Print and shaded views of the part. All mm, measured from the part's lowest x, y and z. Give positions to 0.01 mm unless a question says otherwise; leave off trailing zeros. Loops run counter-clockwise (first coordinate to the right, second up) from the corner with the lowest first, then second, coordinate; pieces in that order, holes last. Notation, with made-up numbers: (78, 34) - (116, 34) arc R19 ccw to (116, 50) - close; hole circle Ø2 at (34, 61). An arc over 180 degrees is marked (long way). Return JSON: item names as keys, results as strings.
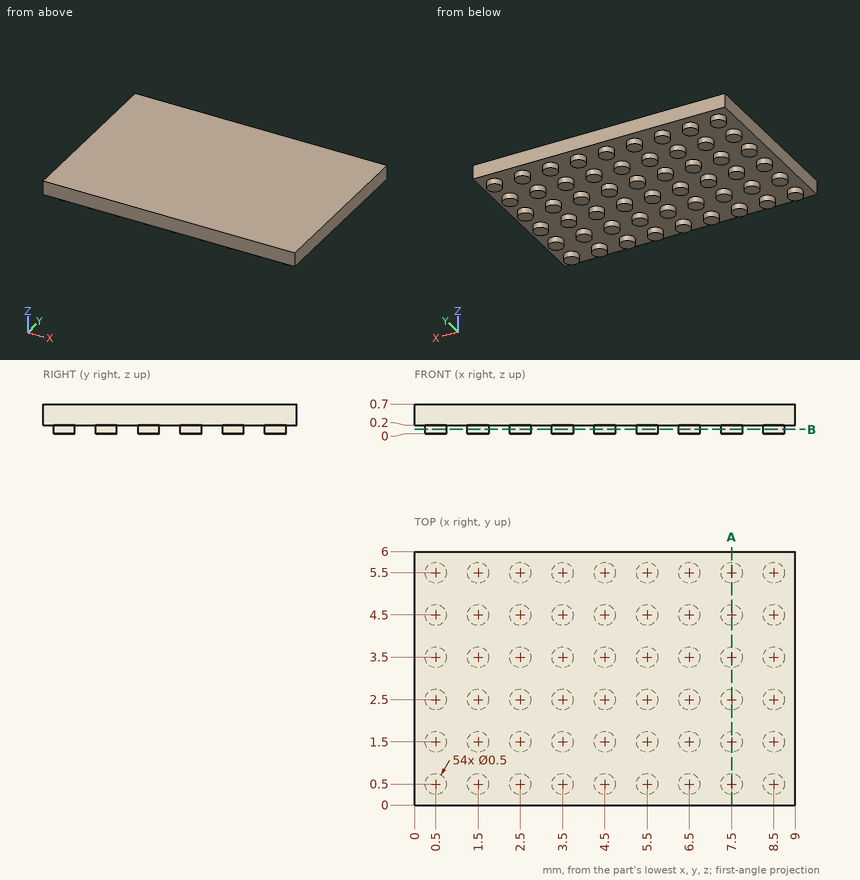
1. Cut at B-B, the plane z = 0.1. Give the number of separate pieces and of enclosed holes in the cut face, plus the area to 3 significant figures.
Values follow:
{"separate pieces": "54", "enclosed holes": "0", "area": "10.6 mm²"}
2. Drill centre lines: probe 1 along Y at (x, z) = (0.5, 0.1); probe 2 along Z at (x, y) = (5, 5.5). Where is each one in solid material? Low to high.
Values follow:
{"probe 1": "y = 0.25 to 0.75, 1.25 to 1.75, 2.25 to 2.75, 3.25 to 3.75, 4.25 to 4.75, 5.25 to 5.75", "probe 2": "z = 0.2 to 0.7"}
3. Cut at A-A, the plane x = 7.5. Write the cut outline in (y, z), plus the area to 3 significant figures.
Values follow:
{"outline": "(0, 0.2) - (0.25, 0.2) - (0.25, 0) - (0.75, 0) - (0.75, 0.2) - (1.25, 0.2) - (1.25, 0) - (1.75, 0) - (1.75, 0.2) - (2.25, 0.2) - (2.25, 0) - (2.75, 0) - (2.75, 0.2) - (3.25, 0.2) - (3.25, 0) - (3.75, 0) - (3.75, 0.2) - (4.25, 0.2) - (4.25, 0) - (4.75, 0) - (4.75, 0.2) - (5.25, 0.2) - (5.25, 0) - (5.75, 0) - (5.75, 0.2) - (6, 0.2) - (6, 0.7) - (0, 0.7) - close", "area": "3.60 mm²"}
